The model under review builds one solid part; all positions refer to its coordinate system, in mm. Round coordinates to 2 decimals unless told otherwise and drop trailing zeros. Loops run counter-clockwise (first coordinate to the right, second up) from the corner with the lowest first, then second, coordinate; pieces in that order, holes last. Notation, with made-up numbers: M 5,-34.5 L 17,-34.5 A18 cw 17,-30.5 Z; hole C -11.75,49 d9. An arc over 180 degrees is marked long. Answer in a Markdown table with one row per item. Add a question column.
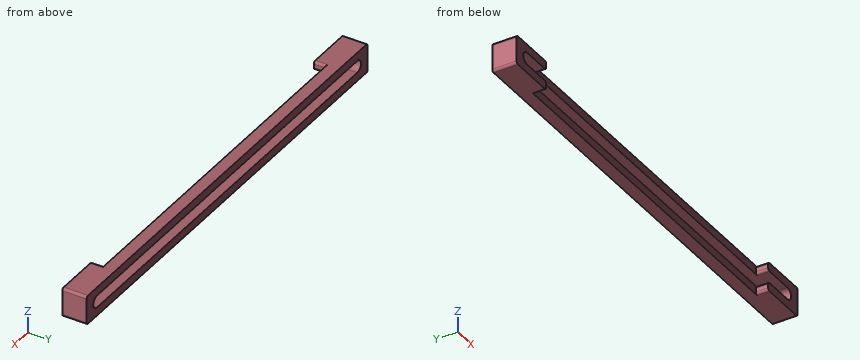
from build123d import *

# Parameters (mm, degrees)
ESQUISSE1_W        = 190
ESQUISSE1_H        = 12
BOSS_EXTRU_1_DEPTH = 2.5
BOSS_EXTRU_3_DEPTH = 5.1
CONG_1_R           = 1


with BuildPart() as part:
    # Esquisse1 → Boss.-Extru.1 (new body, symmetric)
    with BuildSketch(Plane(origin=(0, 0, 0), x_dir=(1, 0, 0), z_dir=(0, 1, 0))):
        Rectangle(ESQUISSE1_W, ESQUISSE1_H)
        with BuildLine():
            Line((-88, 2.5), (88, 2.5))
            ThreePointArc((88, 2.5), (90.5, 0), (88, -2.5))
            Line((88, -2.5), (-88, -2.5))
            ThreePointArc((-88, -2.5), (-90.5, 0), (-88, 2.5))
        make_face(mode=Mode.SUBTRACT)
    extrude(amount=BOSS_EXTRU_1_DEPTH, both=True)

    # Esquisse4 → Boss.-Extru.3 (add)
    with BuildSketch(Plane.XZ.offset(2.5)):
        with BuildLine():
            Line((-95, 6), (-75, 6))
            Line((-75, 6), (-75, 2.5))
            Line((-75, 2.5), (-88, 2.5))
            ThreePointArc((-88, 2.5), (-90.5, 0), (-88, -2.5))
            Line((-88, -2.5), (-75, -2.5))
            Line((-75, -2.5), (-75, -6))
            Line((-75, -6), (-95, -6))
            Line((-95, -6), (-95, 6))
        make_face()
    boss_extru_3 = extrude(amount=BOSS_EXTRU_3_DEPTH)

    # Symétrie2: Boss.-Extru.3 across plane
    add(boss_extru_3.mirror(Plane(origin=(0, 0, 0), x_dir=(0, 0, 1), z_dir=(1, 0, 0))))

    # Congé1
    cong_1_edges = [part.edges().sort_by_distance(p)[0] for p in [
        (-75, -5.05, -6),
        (-75, -5.05, -2.5),
        (-75, -5.05, 2.5),
        (-75, -5.05, 6),
        (75, -5.05, 6),
        (75, -5.05, 2.5),
        (75, -5.05, -2.5),
        (75, -5.05, -6),
        (95, -2.55, 6),
        (-95, -2.55, 6),
        (-95, -2.55, -6),
        (95, -2.55, -6),
    ]]
    fillet(cong_1_edges, radius=CONG_1_R)


solid = part.part
1. Take a section at C-C, the plane z = 0.75. State the section outline as (x, y) points.
2. Take a section at A-A, the plane x = 83. State the section outline as (y, z) points, and give its area (3 significant figures).
3. For pin 1 Ø3 at (x, z) = (-34, -5) entering from -Y, flat-tipped, find the tip position at first contact; note if it passes through.
4. Take a section at B-B, the plane y = -0.75. State the section outline as (x, z) points.
5. To check wall thickness, follow probe 1 along X at (y, z) = (-5.5, 3.5); probe 2 along Z at (x, y) = (87.5, -2.5); probe 3 along Y at (x, z) = (22, -3.25). State the ranges of each line that lie inside material, in increasing order.
Check sheet entries:
| question | item | result |
|---|---|---|
| 1 | outline | M -95,-7.6 L -90.38,-7.6 L -90.38,2.5 L -95,2.5 Z; M 90.38,-7.6 L 95,-7.6 L 95,2.5 L 90.38,2.5 Z |
| 2 | outline | M -7.6,-6 L 2.5,-6 L 2.5,-2.5 L -7.6,-2.5 Z; M -7.6,2.5 L 2.5,2.5 L 2.5,6 L -7.6,6 Z |
| 2 | area | 70.7 mm^2 |
| 3 | pin 1 | stops at y = -2.5 |
| 4 | outline | M -95,-5 A1 ccw -94,-6 L 94,-6 A1 ccw 95,-5 L 95,5 A1 ccw 94,6 L -94,6 A1 ccw -95,5 Z; hole M -88,-2.5 L 88,-2.5 A2.5 ccw 88,2.5 L -88,2.5 A2.5 ccw Z |
| 5 | probe 1 | x = -95 to -75, 75 to 95 |
| 5 | probe 2 | z = -6 to -2.5, 2.5 to 6 |
| 5 | probe 3 | y = -2.5 to 2.5 |
